from build123d import *

# Parameters (mm, degrees)
EXTRUDE013_DEPTH = 2
SKETCH002_R      = 3.5
SKETCH002_R_2    = 1.6
EXTRUDE002_DEPTH = 4.1
SKETCH003_R      = 1.6
EXTRUDE003_DEPTH = 1.6
EXTRUDE008_DEPTH = 4
EXTRUDE001_DEPTH = 5.7
SKETCH_R         = 1.6
EXTRUDE_DEPTH    = 2


with BuildPart() as extrude013:
    # Sketch013 (on Face1 of Fusion) → Extrude013 (new body)
    with BuildSketch(Plane(origin=(0, 0, 0), x_dir=(1, 0, 0), z_dir=(0, 0, -1))):
        Polygon((6.484679, -9.55), (6.484679, -6.45), (3.8, -4.9), (1.115321, -6.45), (1.115321, -9.55), (3.8, -11.1), align=None)
        Polygon((68.16, -11.1), (70.844679, -9.55), (70.844679, -6.45), (68.16, -4.9), (65.475321, -6.45), (65.475321, -9.55), align=None)
        Polygon((61.524679, -53.2), (58.84, -51.65), (56.155321, -53.2), (56.155321, -56.3), (58.84, -57.85), (61.524679, -56.3), align=None)
        Polygon((25.324679, -53.2), (22.64, -51.65), (19.955321, -53.2), (19.955321, -56.3), (22.64, -57.85), (25.324679, -56.3), align=None)
    extrude(amount=-EXTRUDE013_DEPTH)


with BuildPart() as extrude002:
    # Sketch002 (on Face12 of Extrude) → Extrude002 (new body)
    with BuildSketch(Plane.XY.offset(2)):
        with Locations((22.64, 54.75)):
            Circle(SKETCH002_R)
        with Locations((22.64, 54.75)):
            Circle(SKETCH002_R_2, mode=Mode.SUBTRACT)
        with Locations((58.84, 54.75)):
            Circle(SKETCH002_R)
        with Locations((58.84, 54.75)):
            Circle(SKETCH002_R_2, mode=Mode.SUBTRACT)
        with BuildLine():
            ThreePointArc((6.672281, 6), (6.357658, 10.389223), (2, 11.001666))
            Line((2, 4), (2, 11.001666))
            Line((2, 4), (69.96, 4))
            Line((69.96, 4), (69.96, 11.001666))
            ThreePointArc((69.96, 11.001666), (65.602342, 10.389223), (65.287719, 6))
            Line((65.287719, 6), (6.672281, 6))
        make_face()
        with Locations((3.8, 8)):
            Circle(SKETCH002_R_2, mode=Mode.SUBTRACT)
        with Locations((68.16, 8)):
            Circle(SKETCH002_R_2, mode=Mode.SUBTRACT)
    extrude(amount=EXTRUDE002_DEPTH)


with BuildPart() as extrude003:
    # Sketch003 (on Face10 of Extrude002) → Extrude003 (new body)
    with BuildSketch(Plane.XY.offset(6.1)):
        with BuildLine():
            Line((66.55, 4), (69.96, 4))
            Line((69.96, 4), (69.96, 11.001666))
            ThreePointArc((69.96, 11.001666), (68.268796, 11.498309), (66.55, 11.107716))
            Line((66.55, 11.107716), (66.55, 4))
        make_face()
        with Locations((68.16, 8)):
            Circle(SKETCH003_R, mode=Mode.SUBTRACT)
        with BuildLine():
            ThreePointArc((5.41, 11.107716), (3.691204, 11.498309), (2, 11.001666))
            Line((2, 11.001666), (2, 4))
            Line((2, 4), (5.41, 4))
            Line((5.41, 11.107716), (5.41, 4))
        make_face()
        with Locations((3.8, 8)):
            Circle(SKETCH003_R, mode=Mode.SUBTRACT)
    extrude(amount=EXTRUDE003_DEPTH)


with BuildPart() as extrude008:
    # Sketch008 (on Face9 of Extrude001) → Extrude008 (new body)
    with BuildSketch(Plane(origin=(0, 61.42, 0), x_dir=(-1, 0, 0), z_dir=(0, 1, 0))):
        with BuildLine():
            ThreePointArc((-13.683863, 7.7), (-11.21, 4.3), (-8.736137, 7.7))
            Line((-13.683863, 7.7), (-8.736137, 7.7))
        make_face()
    extrude(amount=-EXTRUDE008_DEPTH)


with BuildPart() as cut:
    # Sketch001 (on Face12 of Extrude) → Extrude001 (new body)
    with BuildSketch(Plane.XY.offset(2)):
        with BuildLine():
            Line((0, 0), (0, 60.42))
            ThreePointArc((1, 61.42), (0.292893, 61.127107), (0, 60.42))
            Line((1, 61.42), (70.96, 61.42))
            ThreePointArc((71.96, 60.42), (71.667107, 61.127107), (70.96, 61.42))
            Line((71.96, 60.42), (71.96, 0))
            Line((71.96, 0), (69.96, 0))
            Line((69.96, 0), (69.96, 59.42))
            Line((69.96, 59.42), (2, 59.42))
            Line((2, 59.42), (2, 0))
            Line((2, 0), (0, 0))
        make_face()
    extrude(amount=EXTRUDE001_DEPTH)

    # Cut: cut Extrude008
    add(extrude008.part, mode=Mode.SUBTRACT)


with BuildPart() as cut005:
    # Sketch → Extrude (new body)
    with BuildSketch(Plane.XY):
        with BuildLine():
            Line((0, 0), (71.96, 0))
            Line((71.96, 0), (71.96, 60.42))
            ThreePointArc((71.96, 60.42), (71.667107, 61.127107), (70.96, 61.42))
            Line((70.96, 61.42), (1, 61.42))
            ThreePointArc((1, 61.42), (0.292893, 61.127107), (0, 60.42))
            Line((0, 60.42), (0, 0))
        make_face()
        with Locations((22.64, 54.75)):
            Circle(SKETCH_R, mode=Mode.SUBTRACT)
        with Locations((58.84, 54.75)):
            Circle(SKETCH_R, mode=Mode.SUBTRACT)
        with Locations((3.8, 8)):
            Circle(SKETCH_R, mode=Mode.SUBTRACT)
        with Locations((68.16, 8)):
            Circle(SKETCH_R, mode=Mode.SUBTRACT)
    extrude(amount=EXTRUDE_DEPTH)

    # Fusion: union Extrude002, Extrude003, Cut
    add(extrude002.part)
    add(extrude003.part)
    add(cut.part)

    # Cut005: cut Extrude013
    add(extrude013.part, mode=Mode.SUBTRACT)


solid = cut005.part
Work out the finished part from the listing and answer in its coordinate system (mm). A direction names the side the tool comes from. Coordinates: 2 decimals unless noted, no trailing zeros. Write each loop counter-clockwise with the first axis right and the second up, starting at its lowest first coordinate (ties: lowest second). Pieces come first, ordered by that corner, then holes. Notation, with made-up numbers: M -2.75,-13 L 48.25,-13 A31 ccw 48.25,15 Z; hole C 19.25,11 d6. An arc over 180 degrees is marked long. Use one line per item in the form item = value. Start each with the question number.
1. The part is cut by section B-B (z = 3.5). Give the vertices of the cut face in (x, y), plus the area to 3 significant figures.
2. The part is cut by section D-D (x = 45). Give the vertices of the cut face in (y, z), plus the area to 3 significant figures.
3. The part is cut by section A-A (z = 6.9). Give the vertices of the cut face in (x, y).
4. The mould has two halves that part along Y. Classify faces 6 (the face through (2, 36, 5)), 7 (the face through (36.1, 0, 1.6)), 8 (the face through (11.3, 60.4, 4.3)): released by +Y, released by -Y, zero draft, split by the parting line, or undercut.
5. Each of these flat-tipped pins is pushed along its axis until it touches: P1, Ø1.5, axis at x = 22.5, z = 7, coming from the -Y side; P2, Ø1.5, axis at x = 54, z = 6.5, coming from the -Y side; P3, Ø2.5, axis at x = 58.84, y = 54.75, coming from the +Z side. Where does it stop, or does it pass through?
6. A tool of negligible diameter and unlimited length cuts with its end or side. For faces 1 (the face through (20.06, 57.115, 4.021)), 2 (the face through (66.56, 8.07, 4.81)), 3 (the face through (36, 2, 2)), 4 (the face through (57.479, 57.064, 0.986)), 5 (the face through (71, 42, 7.7)), from which of +Z, -Z, +X, -X, +Y, -Y can it reach the whole face along a straight path? Write none if from no direction.
7. The part is cut by section C-C (y = 8). Give the number of separate pieces and of enclosed holes in the cut face, plus the area to 3 significant figures.
8. Straight lines are drawn through the part: probe 1 along Y at (x, z) = (3.8, 6.5); probe 2 along X at (y, z) = (8, 4.6); probe 3 along X at (y, z) = (9, 3.5). For each, find the intervals that lie inside material, in ascending order. Write a range as from..to.
Evaluation:
q1.outline = M 0,0 L 2,0 L 2,4 L 69.96,4 L 69.96,0 L 71.96,0 L 71.96,60.42 A1 ccw 70.96,61.42 L 1,61.42 A1 ccw 0,60.42 Z; C 22.64,54.75 d7; C 58.84,54.75 d7; hole M 2,11 A3.5 cw 6.67,6 L 65.29,6 A3.5 cw 69.96,11 L 69.96,59.42 L 2,59.42 Z; hole C 3.8,8 d3.2; hole C 22.64,54.75 d3.2; hole C 58.84,54.75 d3.2; hole C 68.16,8 d3.2
q1.area = 614 mm^2
q2.outline = M 0,0 L 61.42,0 L 61.42,7.7 L 59.42,7.7 L 59.42,2 L 6,2 L 6,6.1 L 4,6.1 L 4,2 L 0,2 Z
q2.area = 142 mm^2
q3.outline = M 0,0 L 2,0 L 2,4 L 5.41,4 L 5.41,11.11 A3.5 ccw 2,11 L 2,59.42 L 8.61,59.42 L 8.61,61.42 L 1,61.42 A1 ccw 0,60.42 Z; M 13.81,59.42 L 69.96,59.42 L 69.96,11 A3.5 ccw 66.55,11.11 L 66.55,4 L 69.96,4 L 69.96,0 L 71.96,0 L 71.96,60.42 A1 ccw 70.96,61.42 L 13.81,61.42 Z; hole C 3.8,8 d3.2; hole C 68.16,8 d3.2
q4.face_6 = undercut
q4.face_7 = released by -Y
q4.face_8 = zero draft
q5.P1 = 59.42
q5.P2 = 4
q5.P3 = through
q6.face_1 = +Z
q6.face_2 = +Z, -Z
q6.face_3 = +Z, -Y
q6.face_4 = -Z
q6.face_5 = +Z, +X, -X, +Y, -Y
q7.separate_pieces = 3
q7.enclosed_holes = 0
q7.area = 163 mm^2
q8.probe_1 = 4..6.4, 9.6..11.5, 59.42..61.42
q8.probe_2 = 0..2.2, 5.4..7.3, 64.66..66.56, 69.76..71.96
q8.probe_3 = 0..2.55, 5.05..7.15, 64.81..66.91, 69.41..71.96
